Can you work these out from the model? Positions are in its coordinate system, mm. A direction names the side the tool comes from. Give positions to 0.01 mm unless a question says otherwise; leave off trailing zeros. Order: outer loops, then holes, each group sorted by start corner. A loop starts at its lowest first (then second) coordinate and runs counter-clockwise, first axis right, second up.
```python
from build123d import *

# Parameters (mm, degrees)
SKETCH2_R           = 76.2
BOSS_EXTRUDE1_DEPTH = 6.35
SKETCH3_R           = 73.025
BOSS_EXTRUDE2_DEPTH = 9.525
SKETCH4_R           = 69.85
BOSS_EXTRUDE3_DEPTH = 15.875
SKETCH6_R           = 73.025
BOSS_EXTRUDE4_DEPTH = 3.175
SKETCH7_R           = 69.85
BOSS_EXTRUDE5_DEPTH = 6.35
SKETCH8_R           = 73.025
BOSS_EXTRUDE6_DEPTH = 6.35
SKETCH9_R           = 66.675
CUT_EXTRUDE1_DEPTH  = 113.342968182
SKETCH10_R          = 0.79375
CUT_EXTRUDE2_DEPTH  = 111.716033166
SKETCH11_R          = 73.025
SKETCH11_R_2        = 69.85
CUT_EXTRUDE3_DEPTH  = 3.175
SKETCH12_R          = 0.79375
CUT_EXTRUDE4_DEPTH  = 3.175


with BuildPart() as part:
    # Sketch2 → Boss-Extrude1 (new body)
    with BuildSketch(Plane(origin=(0, 0, 0), x_dir=(1, 0, 0), z_dir=(0, 1, 0))):
        with Locations(Location((0, 0, 0), (0, 0, 270))):
            Circle(SKETCH2_R)
    extrude(amount=BOSS_EXTRUDE1_DEPTH)

    # Sketch3 → Boss-Extrude2 (add)
    with BuildSketch(Plane(origin=(0, 0, 0), x_dir=(1, 0, 0), z_dir=(0, 1, 0))):
        with Locations(Location((0, 0, 0), (0, 0, 90))):
            Circle(SKETCH3_R)
    extrude(amount=BOSS_EXTRUDE2_DEPTH)

    # Sketch4 → Boss-Extrude3 (add)
    with BuildSketch(Plane(origin=(0, 0, 0), x_dir=(1, 0, 0), z_dir=(0, 1, 0))):
        with Locations(Location((0, 0, 0), (0, 0, 270))):
            Circle(SKETCH4_R)
    extrude(amount=BOSS_EXTRUDE3_DEPTH)

    # Sketch6 → Boss-Extrude4 (add)
    with BuildSketch(Plane(origin=(0, 15.875, 0), x_dir=(1, 0, 0), z_dir=(0, 1, 0))):
        with Locations(Location((0, 0, 0), (0, 0, 90))):
            Circle(SKETCH6_R)
    extrude(amount=BOSS_EXTRUDE4_DEPTH)

    # Sketch7 → Boss-Extrude5 (add)
    with BuildSketch(Plane(origin=(0, 19.05, 0), x_dir=(1, 0, 0), z_dir=(0, 1, 0))):
        with Locations(Location((0, 0, 0), (0, 0, 270))):
            Circle(SKETCH7_R)
    extrude(amount=BOSS_EXTRUDE5_DEPTH)

    # Sketch8 → Boss-Extrude6 (add)
    with BuildSketch(Plane(origin=(0, 25.4, 0), x_dir=(1, 0, 0), z_dir=(0, 1, 0))):
        with Locations(Location((0, 0, 0), (0, 0, 90))):
            Circle(SKETCH8_R)
    extrude(amount=BOSS_EXTRUDE6_DEPTH)

    # Sketch9 → Cut-Extrude1 (cut, through all)
    with BuildSketch(Plane.XZ):
        with Locations(Location((0, 0, 0), (0, 0, 270))):
            Circle(SKETCH9_R)
    extrude(amount=-CUT_EXTRUDE1_DEPTH, mode=Mode.SUBTRACT)

    # Sketch10 → Cut-Extrude2 (cut, through all)
    with BuildSketch(Plane(origin=(0, 6.35, 0), x_dir=(1, 0, 0), z_dir=(0, 1, 0))):
        with Locations(Location((0, 74.6125, 0), (0, 0, 270))):
            Circle(SKETCH10_R)
        with Locations(Location((52.759004711, 52.759004711, 0), (0, 0, 270))):
            Circle(SKETCH10_R)
        with Locations(Location((74.6125, 0, 0), (0, 0, 270))):
            Circle(SKETCH10_R)
        with Locations(Location((52.759004711, -52.759004711, 0), (0, 0, 270))):
            Circle(SKETCH10_R)
        with Locations(Location((0, -74.6125, 0), (0, 0, 270))):
            Circle(SKETCH10_R)
        with Locations(Location((-52.759004711, -52.759004711, 0), (0, 0, 270))):
            Circle(SKETCH10_R)
        with Locations(Location((-74.6125, 0, 0), (0, 0, 270))):
            Circle(SKETCH10_R)
        with Locations(Location((-52.759004711, 52.759004711, 0), (0, 0, 270))):
            Circle(SKETCH10_R)
    extrude(amount=-CUT_EXTRUDE2_DEPTH, mode=Mode.SUBTRACT)

    # Sketch11 → Cut-Extrude3 (cut)
    with BuildSketch(Plane.XZ):
        with Locations(Location((0, 0, 0), (0, 0, 270))):
            Circle(SKETCH11_R)
        with Locations(Location((0, 0, 0), (0, 0, 90))):
            Circle(SKETCH11_R_2, mode=Mode.SUBTRACT)
    extrude(amount=-CUT_EXTRUDE3_DEPTH, mode=Mode.SUBTRACT)

    # Sketch12 → Cut-Extrude4 (cut)
    with BuildSketch(Plane(origin=(0, 31.75, 0), x_dir=(1, 0, 0), z_dir=(0, 1, 0))):
        with Locations(Location((0, -69.85, 0), (0, 0, 270))):
            Circle(SKETCH12_R)
        with Locations(Location((-69.85, 0, 0), (0, 0, 270))):
            Circle(SKETCH12_R)
        with Locations(Location((0, 69.85, 0), (0, 0, 270))):
            Circle(SKETCH12_R)
        with Locations(Location((69.85, 0, 0), (0, 0, 270))):
            Circle(SKETCH12_R)
    extrude(amount=-CUT_EXTRUDE4_DEPTH, mode=Mode.SUBTRACT)


solid = part.part
```
1) Which directions (+Z, -Z, +X, -X, +Y, -Y) give clear straight access to the entire face, cutting with the end or side of a thin tool? Please do faces 1 (the face through (-62, 0, 39)), 2 (the face through (16, 31.75, 65)), 3 (the face through (-62, 6.35, 39)), 4 (the face through (21.935, 1.565, -69.653)), 5 (the face through (38, 9.525, -59)).
2) I'm going to push flat-ended pins straight in: pin 1 Ø1 at (x, y) = (45, 17) entering from -Z; pin 2 Ø1.4 at (x, z) = (-52.76, -52.76) entering from -Y; pin 3 Ø3 at (y, z) = (3.5, 6.5) entering from -X; pin 4 Ø12 at (x, y) = (33.5, 24) entering from +Z. Where does each tip first touch, or does it pass through?
3) If I drill on line 1 (Y direction, x = 54, z = -48) (3 decimals); line 2 (X direction, y = 3, z = 0) (3 decimals); line 3 (Z direction, x = -31.5, y = 2), over which ranges is the centre line in solid material (lowest first)?
4) Suppose I cut it at A-A (y = 11.5). Please give me the cut outline in (x, z) (3 decimals), and give its area (3 significant figures).
5) We'd pull the mould along Z, two halves only. Please class faces 6 (the face through (-68.2, 22.2, -15.1)), 7 (the face through (68.2, 1.6, -15.1)), 8 (the face through (38, 19.05, -59)): +Z half, -Z half, draft (parallel to the pull), parting line (faces both ways), or undercut.
Results:
1. face 1: +Z, -Z, +X, -X, -Y
1. face 2: +Z, -Z, +X, -X, +Y
1. face 3: +Y
1. face 4: -Y
1. face 5: none
2. pin 1: stops at z = -57.9
2. pin 2: passes through
2. pin 3: stops at x = -76.04
2. pin 4: stops at z = 67.58
3. line 1: y = 3.175 to 9.525, 15.875 to 19.05, 25.4 to 31.75
3. line 2: x = -76.2 to -75.406, -73.819 to -73.025, -69.85 to -66.675, 66.675 to 69.85, 73.025 to 73.819, 75.406 to 76.2
3. line 3: z = -69.38 to -65.88, -62.34 to -58.76, 58.76 to 62.34, 65.88 to 69.38
4. outline: circle Ø139.7 at (0, 0); hole circle Ø133.35 at (0, 0)
4. area: 1,360 mm2
5. face 6: parting line
5. face 7: undercut
5. face 8: draft
